Verification items for the finished model (mm, model axes). Face numbers are marked on the shaded views. A direction names the side the tool comes from. Give positions to 0.01 mm unless a question says otherwise; leave off trailing zeros. Order: outer loops, then holes, each group sorted by start corner. A loop starts at its lowest first (then second) coordinate and runs counter-clockwise, first axis right, second up. Notation, with made-up numbers: (-10, 72.25) -> (22, 72.25) arc R25 cw to (22, 108.25) -> close; hole circle Ø8 at (18.5, 40). An arc over 180 degrees is marked (long way). Return JSON: item names as keys, results as strings. Group by question number.
(1) Thickness scan on line 1 along X through (y, z) = (175.69, -10.5); line 2 along Y through (x, z) = (99.69, -9); line 3 along Y through (x, z) = (101.5, -9.8). Record the ranges inside material, lowest first.
(2) Cross-section at A-A on z = -8.9. Enter the section's corners in (x, y), then the cut area to 3 significant figures.
(3) Cross-section at C-C on y = 175.69. Enter the section's corners in (x, z), then the cut area to 3 significant figures.
(4) Cross-section at B-B on x = 99.69. Enter the section's corners in (y, z), then the cut area to 3 significant figures.
(5) Tool access check on the marked faces 5, 6 and 7. Record the directions out of +Z, -Z, +X, -X, +Y, -Y that give a thin tool (end or side, any length) a straight path to the whole face; none if there is none.
(6) Cross-section at D-D on y = 179.5. Enter the section's corners in (x, z), then the cut area to 3 significant figures.
(7) Depth check by flat-ended pin: pin 1 Ø2.5 at (x, z) = (100.5, -9.5) entering from +Y; pin 2 Ø1.5 at (x, z) = (72.5, -11.5) entering from -Y; pin 3 Ø1.5 at (y, z) = (168.5, -9) entering from -X; pin 4 Ø10 at (x, y) = (86.69, 175.69) entering from -Z. Enter the tip coordinate at first touch or a pass-through.
(8) Release check for a two-part mould opening along Y. For the marked faces 1, 2, 3 and 4 record: pulls with the +Y half, pulls with the -Y half, needs draft (parallel to the pull), parting line crosses it, or undercut.
from build123d import *

# Parameters (mm, degrees)
CYLINDER115_R     = 1.5
CYLINDER115_DEPTH = 11
CYLINDER113_R     = 5.5
CYLINDER113_DEPTH = 46
CYLINDER114_R     = 1.5
CYLINDER114_DEPTH = 11
BOX019_W          = 32
BOX019_H          = 10
BOX019_DEPTH      = 5
CYLINDER112_R     = 10
CYLINDER112_DEPTH = 5
CYLINDER111_R     = 7
CYLINDER111_DEPTH = 5


with BuildPart() as obj1:
    # Cylinder115 → Cylinder115 (new body)
    with BuildSketch(Plane(origin=(99.69, 175.69, -10), x_dir=(1, 0, 0), z_dir=(0, 0, 1))):
        Circle(CYLINDER115_R)
    extrude(amount=CYLINDER115_DEPTH)


with BuildPart() as obj2:
    # Cylinder113 → Cylinder113 (new body)
    with BuildSketch(Plane(origin=(86.69, 175.69, -14), x_dir=(1, 0, 0), z_dir=(0, 0, 1))):
        Circle(CYLINDER113_R)
    extrude(amount=CYLINDER113_DEPTH)


with BuildPart() as fusion049:
    # Cylinder114 → Cylinder114 (new body)
    with BuildSketch(Plane(origin=(73.69, 175.69, -10), x_dir=(1, 0, 0), z_dir=(0, 0, 1))):
        Circle(CYLINDER114_R)
    extrude(amount=CYLINDER114_DEPTH)

    # Fusion049: union obj1, obj2
    add(obj1.part)
    add(obj2.part)


with BuildPart() as obj3:
    # Box019 → Box019 (new body)
    with BuildSketch(Plane(origin=(70.69, 170.69, -5), x_dir=(1, 0, 0), z_dir=(0, 0, 1))):
        with Locations((16, 5)):
            Rectangle(BOX019_W, BOX019_H)
    extrude(amount=BOX019_DEPTH)


with BuildPart() as obj4:
    # Cylinder112 → Cylinder112 (new body)
    with BuildSketch(Plane(origin=(86.69, 175.69, -5), x_dir=(1, 0, 0), z_dir=(0, 0, 1))):
        Circle(CYLINDER112_R)
    extrude(amount=CYLINDER112_DEPTH)


with BuildPart() as obj5:
    # Cylinder111 → Cylinder111 (new body)
    with BuildSketch(Plane(origin=(86.69, 175.69, -5), x_dir=(1, 0, 0), z_dir=(0, 0, 1))):
        Circle(CYLINDER111_R)
    extrude(amount=CYLINDER111_DEPTH)

    # Fusion048: union obj3, obj4
    add(obj3.part)
    add(obj4.part)

    # Cut014: cut Fusion049
    add(fusion049.part, mode=Mode.SUBTRACT)


with BuildPart() as obj5_1:
    # Cut014 placement: moved
    add(obj5.part.moved(Location((0, 0, -8))))


solid = obj5_1.part
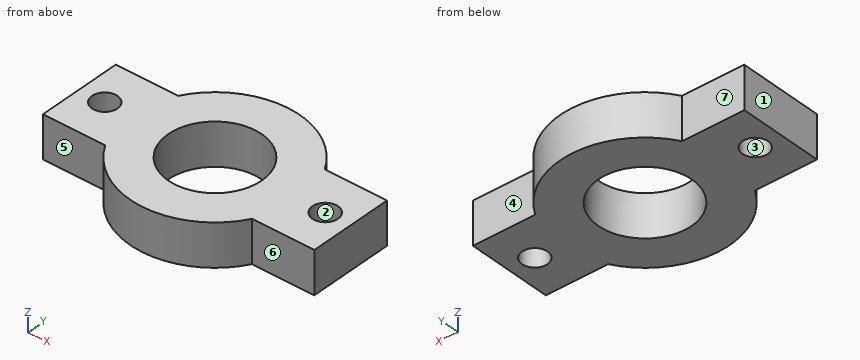
Verdict:
{
 "1": {"line 1": "70.69 to 72.19, 75.19 to 81.19, 92.19 to 98.19, 101.19 to 102.69", "line 2": "170.69 to 174.19, 177.19 to 180.69", "line 3": "170.69 to 180.69"},
 "2": {"outline": "(70.69, 170.69) -> (78.03, 170.69) arc R10 ccw to (95.35, 170.69) -> (102.69, 170.69) -> (102.69, 180.69) -> (95.35, 180.69) arc R10 ccw to (78.03, 180.69) -> (70.69, 180.69) -> close; hole circle Ø3 at (73.69, 175.69); hole circle Ø11 at (86.69, 175.69); hole circle Ø3 at (99.69, 175.69)", "area": "334 mm²"},
 "3": {"outline": "(70.69, -13) -> (72.19, -13) -> (72.19, -8) -> (70.69, -8) -> close; (75.19, -13) -> (81.19, -13) -> (81.19, -8) -> (75.19, -8) -> close; (92.19, -13) -> (98.19, -13) -> (98.19, -8) -> (92.19, -8) -> close; (101.19, -13) -> (102.69, -13) -> (102.69, -8) -> (101.19, -8) -> close", "area": "75.0 mm²"},
 "4": {"outline": "(170.69, -13) -> (174.19, -13) -> (174.19, -8) -> (170.69, -8) -> close; (177.19, -13) -> (180.69, -13) -> (180.69, -8) -> (177.19, -8) -> close", "area": "35.0 mm²"},
 "5": {"face 5": "+Z, -Z, -X, -Y", "face 6": "+Z, -Z, +X, -Y", "face 7": "+Z, -Z, -X, +Y"},
 "6": {"outline": "(70.69, -13) -> (82.72, -13) -> (82.72, -8) -> (70.69, -8) -> close; (90.66, -13) -> (102.69, -13) -> (102.69, -8) -> (90.66, -8) -> close", "area": "120 mm²"},
 "7": {"pin 1": "y = 180.69", "pin 2": "y = 170.69", "pin 3": "x = 79.04", "pin 4": "through"},
 "8": {"face 1": "needs draft", "face 2": "undercut", "face 3": "undercut", "face 4": "pulls with the +Y half"}
}
